from build123d import *

# Parameters (mm, degrees)
SKETCH2_W           = 190.5
SKETCH2_H           = 203.2
BOSS_EXTRUDE1_DEPTH = 6
SKETCH3_R           = 2
CUT_EXTRUDE2_DEPTH  = 6
CUT_EXTRUDE3_DEPTH  = 7
SKETCH5_R           = 2.5
CUT_EXTRUDE6_DEPTH  = 7
CUT_EXTRUDE12_DEPTH = 10
CUT_EXTRUDE13_DEPTH = 7


with BuildPart() as part:
    # Sketch2 → Boss-Extrude1 (new body)
    with BuildSketch(Plane(origin=(0, 0, 0), x_dir=(1, 0, 0), z_dir=(0, 1, 0))):
        Rectangle(SKETCH2_W, SKETCH2_H)
    extrude(amount=BOSS_EXTRUDE1_DEPTH)

    # Sketch3 → Cut-Extrude2 (cut)
    with BuildSketch(Plane(origin=(0, 6, 0), x_dir=(1, 0, 0), z_dir=(0, 1, 0))):
        with Locations((-77.47, 34.216206602)):
            Circle(SKETCH3_R)
        with Locations((-77.47, 80.0880034)):
            Circle(SKETCH3_R)
        with Locations((77.47, 34.216206602)):
            Circle(SKETCH3_R)
        with Locations((77.47, 80.0880034)):
            Circle(SKETCH3_R)
        with Locations((-59.69, 80.0880034)):
            Circle(SKETCH3_R)
        with Locations((-59.69, 34.216206602)):
            Circle(SKETCH3_R)
        with Locations((59.69, 80.0880034)):
            Circle(SKETCH3_R)
        with Locations((59.69, 34.216206602)):
            Circle(SKETCH3_R)
    extrude(amount=-CUT_EXTRUDE2_DEPTH, mode=Mode.SUBTRACT)

    # Sketch4 → Cut-Extrude3 (cut, through all)
    with BuildSketch(Plane(origin=(0, 6, 0), x_dir=(1, 0, 0), z_dir=(0, 1, 0))):
        with BuildLine():
            Line((-34.925, -90.199433694), (34.925, -90.199433694))
            ThreePointArc((34.925, -90.199433694), (36.425, -91.699433694), (34.925, -93.199433694))
            Line((34.925, -93.199433694), (-34.925, -93.199433694))
            ThreePointArc((-34.925, -93.199433694), (-36.425, -91.699433694), (-34.925, -90.199433694))
        make_face()
    extrude(amount=-CUT_EXTRUDE3_DEPTH, mode=Mode.SUBTRACT)

    # Sketch5 → Cut-Extrude6 (cut, through all)
    with BuildSketch(Plane(origin=(0, 6, 0), x_dir=(1, 0, 0), z_dir=(0, 1, 0))):
        with Locations((-78.187036158, 94.165073798)):
            Circle(SKETCH5_R)
        with Locations((0, 94.165073798)):
            Circle(SKETCH5_R)
        with Locations((78.187036158, 0)):
            Circle(SKETCH5_R)
        with Locations((0, -80.0880034)):
            Circle(SKETCH5_R)
        with Locations((-78.187036158, 0)):
            Circle(SKETCH5_R)
        with Locations((78.187036158, 94.165073798)):
            Circle(SKETCH5_R)
        with Locations((-78.187036158, -94.165073798)):
            Circle(SKETCH5_R)
        with Locations((78.187036158, -94.165073798)):
            Circle(SKETCH5_R)
    extrude(amount=-CUT_EXTRUDE6_DEPTH, mode=Mode.SUBTRACT)

    # Sketch8 → Cut-Extrude12 (cut)
    with BuildSketch(Plane(origin=(0, 6, 0), x_dir=(1, 0, 0), z_dir=(0, 1, 0))):
        with BuildLine():
            Line((-30, 29.25), (30, 29.25))
            ThreePointArc((30, 29.25), (31.5, 27.75), (30, 26.25))
            Line((30, 26.25), (-30, 26.25))
            ThreePointArc((-30, 26.25), (-31.5, 27.75), (-30, 29.25))
        make_face()
        with BuildLine():
            Line((-30, -26.25), (30, -26.25))
            ThreePointArc((30, -26.25), (31.5, -27.75), (30, -29.25))
            Line((30, -29.25), (-30, -29.25))
            ThreePointArc((-30, -29.25), (-31.5, -27.75), (-30, -26.25))
        make_face()
    extrude(amount=-CUT_EXTRUDE12_DEPTH, mode=Mode.SUBTRACT)

    # Sketch9 → Cut-Extrude13 (cut, through all)
    with BuildSketch(Plane(origin=(0, 6, 0), x_dir=(1, 0, 0), z_dir=(0, 1, 0))):
        with BuildLine():
            ThreePointArc((-14.61, -69.152429333), (-16.024213562, -72.566642895), (-12.61, -71.152429333))
            Line((-12.61, -71.152429333), (-14.61, -71.152429333))
            Line((-14.61, -71.152429333), (-14.61, -69.152429333))
        make_face()
        with BuildLine():
            Line((-14.61, -71.152429333), (-12.61, -71.152429333))
            ThreePointArc((-12.61, -71.152429333), (-13.195786438, -69.73821577), (-14.61, -69.152429333))
            Line((-14.61, -69.152429333), (-14.61, -71.152429333))
        make_face()
        with BuildLine():
            ThreePointArc((14.61, -69.152429333), (13.195786438, -69.73821577), (12.61, -71.152429333))
            Line((12.61, -71.152429333), (14.61, -71.152429333))
            Line((14.61, -71.152429333), (14.61, -69.152429333))
        make_face()
        with BuildLine():
            Line((14.61, -71.152429333), (12.61, -71.152429333))
            ThreePointArc((12.61, -71.152429333), (14.61, -73.152429333), (16.61, -71.152429333))
            ThreePointArc((16.61, -71.152429333), (16.024213562, -69.73821577), (14.61, -69.152429333))
            Line((14.61, -69.152429333), (14.61, -71.152429333))
        make_face()
        with BuildLine():
            ThreePointArc((16.61, -48.112429333), (14.61, -46.112429333), (12.61, -48.112429333))
            Line((12.61, -48.112429333), (14.61, -48.112429333))
            Line((14.61, -48.112429333), (14.61, -50.112429333))
            ThreePointArc((14.61, -50.112429333), (16.024213562, -49.526642895), (16.61, -48.112429333))
        make_face()
        with BuildLine():
            Line((14.61, -48.112429333), (12.61, -48.112429333))
            ThreePointArc((12.61, -48.112429333), (13.195786438, -49.526642895), (14.61, -50.112429333))
            Line((14.61, -50.112429333), (14.61, -48.112429333))
        make_face()
        with BuildLine():
            ThreePointArc((-14.61, -50.112429333), (-13.195786438, -49.526642895), (-12.61, -48.112429333))
            Line((-12.61, -48.112429333), (-14.61, -48.112429333))
            Line((-14.61, -48.112429333), (-14.61, -50.112429333))
        make_face()
        with BuildLine():
            Line((-14.61, -48.112429333), (-12.61, -48.112429333))
            ThreePointArc((-12.61, -48.112429333), (-16.024213562, -46.69821577), (-14.61, -50.112429333))
            Line((-14.61, -50.112429333), (-14.61, -48.112429333))
        make_face()
    extrude(amount=-CUT_EXTRUDE13_DEPTH, mode=Mode.SUBTRACT)


solid = part.part
Geometry check sheet. Reference: the model listing, model coordinates, mm. A direction names the side the tool comes from. Round coordinates to 2 decimals unless told otherwise and drop trailing zeros. Loops run counter-clockwise (first coordinate to the right, second up) from the corner with the lowest first, then second, coordinate; pieces in that order, holes last. Notation, with made-up numbers: (49.5, -39.5) -> (105.5, -39.5) arc R19 cw to (105.5, -21.5) -> close; hole circle Ø5 at (88.5, -12.75). An arc over 180 degrees is marked (long way). Answer as a JSON object with one key per item and string values. Group by question number.
Item 1: Set-up check for faces 1 (the face through (0, 3, -29.25)), 2 (the face through (-95.25, 3, 1)): record each of +Z, -Z, +X, -X, +Y, -Y from which the full face is reachable in a straight line by a thin tool's end or side.
Item 2: Release check for a two-part mould opening along Z. For faces 3 (the face through (0, 3, 93.199)), 4 (the face through (-1, 0, -1)), 5 (the face through (-0.542, 3.042, -91.725)), 6 (the face through (-1, 3, -101.6)) record: pulls with the +Z half, pulls with the -Z half, needs draft (parallel to the pull), parting line crosses it, or undercut.
Item 3: Cross-section at A-A, the plane x = 0. Record the cut outline in (y, z).
Item 4: Thickness scan on line 1 along Z through (x, y) = (59.69, 4.7); line 2 along Z through (x, y) = (25.5, 3.7); line 3 along Z through (x, y) = (15, 2.5). Record the ranges inside material, lowest first.
Item 5: Cross-section at B-B, the plane y = 1.75. Count the separate pieces of the cut face and the enclosed holes in it, plus the area to 3 significant figures.
Determined:
{
 "1": {"face 1": "+Y, -Y", "face 2": "+Z, -Z, -X, +Y, -Y"},
 "2": {"face 3": "undercut", "face 4": "needs draft", "face 5": "undercut", "face 6": "pulls with the -Z half"},
 "3": {"outline": "(0, -101.6) -> (6, -101.6) -> (6, -96.67) -> (0, -96.67) -> close; (0, -91.67) -> (6, -91.67) -> (6, -29.25) -> (0, -29.25) -> close; (0, -26.25) -> (6, -26.25) -> (6, 26.25) -> (0, 26.25) -> close; (0, 29.25) -> (6, 29.25) -> (6, 77.59) -> (0, 77.59) -> close; (0, 82.59) -> (6, 82.59) -> (6, 90.2) -> (0, 90.2) -> close; (0, 93.2) -> (6, 93.2) -> (6, 101.6) -> (0, 101.6) -> close"},
 "4": {"line 1": "z = -101.6 to -82.09, -78.09 to -36.22, -32.22 to 101.6", "line 2": "z = -101.6 to -29.25, -26.25 to 26.25, 29.25 to 90.2, 93.2 to 101.6", "line 3": "z = -101.6 to -29.25, -26.25 to 26.25, 29.25 to 46.15, 50.07 to 69.19, 73.11 to 90.2, 93.2 to 101.6"},
 "5": {"separate pieces": "1", "enclosed holes": "23", "area": "37,800 mm²"}
}
